```python
from build123d import *

# Parameters (mm, degrees)
F0_W     = 25.4
F0_H     = 127
F1_DEPTH = 203.2
F2_SIZE  = 19.05
F4_DEPTH = 406.401
F6_DEPTH = 94.293689


with BuildPart() as f1:
    # F0 (on Front) → F1 (new body, symmetric)
    with BuildSketch(Plane.XZ):
        Rectangle(F0_W, F0_H)
    extrude(amount=F1_DEPTH, both=True)

    # F2
    f2_edges = [f1.edges().sort_by_distance(p)[0] for p in [
        (-12.7, 0, 63.5),
        (-12.7, 0, -63.5),
    ]]
    chamfer(f2_edges, length=F2_SIZE)

    # F3 (on face) → F4 (cut, through all)
    with BuildSketch(Plane.XZ.offset(203.2)):
        with BuildLine():
            ThreePointArc((11.060744, 37.774344), (12.279988, 35.370372), (12.7, 32.707811))
            Line((12.7, 32.707811), (12.7, 60.574245))
            ThreePointArc((12.7, 60.574245), (7.734522, 49.472371), (11.060744, 37.774344))
        make_face()
        with BuildLine():
            ThreePointArc((12.7, 32.707811), (12.205083, 29.823985), (10.776971, 27.270186))
            ThreePointArc((10.776971, 27.270186), (6.784667, 15.709988), (11.117322, 4.272996))
            ThreePointArc((11.117322, 4.272996), (12.291618, 2.278342), (12.7, 0))
            Line((12.7, 0), (12.7, 32.707811))
        make_face()
        with BuildLine():
            Line((12.7, -31.853333), (12.7, 0))
            ThreePointArc((12.7, 0), (12.343759, -2.132292), (11.313729, -4.03298))
            ThreePointArc((11.313729, -4.03298), (7.310588, -15.504261), (11.098474, -27.048409))
            ThreePointArc((11.098474, -27.048409), (12.289076, -29.320934), (12.7, -31.853333))
        make_face()
        with BuildLine():
            Line((12.7, -60.624816), (12.7, -31.853333))
            ThreePointArc((12.7, -31.853333), (11.827932, -35.487574), (9.401646, -38.330346))
            ThreePointArc((9.401646, -38.330346), (4.3012, -50.476153), (12.7, -60.624816))
        make_face()
    extrude(amount=-F4_DEPTH, mode=Mode.SUBTRACT)

    # F5 (on face) → F6 (cut, through all)
    with BuildSketch(Plane(origin=(-28.575, 0, 28.575), x_dir=(0, -1, 0), z_dir=(-0.707107, 0, 0.707107))):
        Polygon((203.2, 53.881537), (-203.2, 53.881537), (-198.709872, 49.391409), (203.2, 49.391409), align=None)
        Polygon((-198.709872, 49.391409), (-203.2, 53.881537), (-203.2, 49.391409), align=None)
        Polygon((-198.709872, 49.391409), (-203.2, 49.391409), (-203.2, -78.467675), (-70.850788, -78.467675), align=None)
    extrude(amount=-F6_DEPTH, mode=Mode.SUBTRACT)


solid = f1.part
```
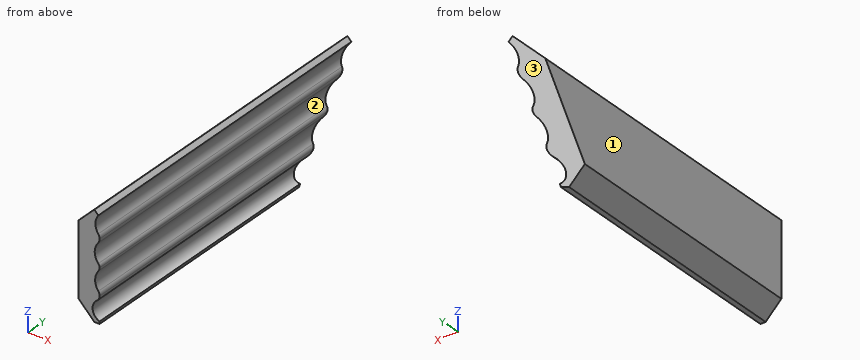
The listing builds one solid part. Answer for the finished solid, in the listing's coordinates (mm). Face numbers are marked on the shaded views. Coordinates: 2 decimals unless noted, no trailing zeros. Write each loop counter-clockwise with the first axis right and the second up, starting at its lowest first coordinate (ties: lowest second). Pieces come first, ordered by that corner, then holes. Notation, with made-up numbers: (22.25, 55.5) - (49.25, 55.5) arc R26 cw to (49.25, 74.5) - close; hole circle Ø9 at (17, -37.5). An arc over 180 degrees is marked (long way). Return JSON: item names as keys, results as strings. Group by question number.
1. Determine the mould class of the marked faces 1, 2 and 3 for opening direction Z: released by +Z, released by -Z, zero draft, split by the parting line, or undercut.
2. A cutting plane is placed at C-C, the plane y = 142. Determine the outline of the cut face in (x, z), plus the area to 3 significant figures.
3. A cutting plane is placed at D-D, the plane x = -2.5. Determine the outline of the cut face in (y, z), plus the area to 3 significant figures.
4. A cutting plane is placed at A-A, the plane y = -25.5. Determine the outline of the cut face in (x, z), plus the area to 3 significant figures.
5. A cutting plane is placed at B-B, the plane z = -15. Determine the outline of the cut face in (x, y).
6. Given pin 1 (12 mm diameter, centred on x = -9, z = 24.5, fed in from +Y); pin 2 (1 mm diameter, centred on x = 4, y = -79, fed in from +Z); pin 3 (4 mm diameter, centred on x = -5, y = 114.5, fed in from +Z), each flat-ended and moving along its own axis, determine where each tip first touches the part or whether it passes through.
7. Straight lines are drawn through the part: L1, parallel to Z at x = 11, y = -138.5; L2, parallel to Z at x = 11.25, y = 30.5; L3, parallel to Z at x = 5.75, y = 166. For each, find the intervals that lie inside material, in ascending order.
Ans:
{
 "1": {"face 1": "zero draft", "face 2": "undercut", "face 3": "released by -Z"},
 "2": {"outline": "(-12.7, 2.35) - (7.43, -17.78) arc R18.95 cw to (11.31, -4.03) arc R6.56 ccw to (12.7, 0) arc R6.56 ccw to (11.12, 4.27) arc R17.97 cw to (10.78, 27.27) arc R8.65 ccw to (11.06, 37.77) arc R17.79 cw to (11.13, 58.72) - (6.35, 63.5) - (-12.7, 44.45) - close", "area": "1,400 mm²"},
 "3": {"outline": "(-203.2, -54.65) - (108.91, -54.65) - (186.19, 54.65) - (-203.2, 54.65) - close", "area": "38,300 mm²"},
 "4": {"outline": "(-12.7, -44.45) - (6.35, -63.5) - (12.7, -63.5) - (12.7, -60.62) arc R12.72 cw to (9.4, -38.33) arc R8.01 ccw to (12.7, -31.85) arc R8.01 ccw to (11.1, -27.05) arc R18.95 cw to (11.31, -4.03) arc R6.56 ccw to (12.7, 0) arc R6.56 ccw to (11.12, 4.27) arc R17.97 cw to (10.78, 27.27) arc R8.65 ccw to (11.06, 37.77) arc R17.79 cw to (11.13, 58.72) - (6.35, 63.5) - (-12.7, 44.45) - close", "area": "2,400 mm²"},
 "5": {"outline": "(-12.7, -203.2) - (7.32, -203.2) - (7.32, 143.89) - (-12.7, 129.73) - close"},
 "6": {"pin 1": "y = 166.28", "pin 2": "z = 61.65", "pin 3": "z = 54.15"},
 "7": {"L1": "-63.5 to -59.89, -36.79 to -26.92, -4.45 to 4.41, 27.56 to 37.86, 58.53 to 58.85", "L2": "-63.5 to -60.02, -36.45 to -27.26, -4.12 to 4.11, 27.91 to 37.5", "L3": "17.84 to 62.9"}
}
